```python
from build123d import *

# Parameters (mm, degrees)
BOSS_EXTRUDE1_DEPTH = 10
FILLET1_R           = 5
FILLET2_R           = 5
FILLET3_R           = 5


# Some blends are built 0.0001 mm under size
with BuildPart() as part:
    # Sketch1 → Boss-Extrude1 (new body)
    with BuildSketch(Plane.XY):
        Polygon((-40, -120.172625832), (-40, 169.827374168), (-25, 169.827374168), (-25, 219.827374168), (5, 219.827374168), (5, -170.172625832), (-25, -170.172625832), (-25, -120.172625832), align=None)
    extrude(amount=BOSS_EXTRUDE1_DEPTH)

    # Fillet1
    fillet1_edges = [part.edges().sort_by_distance(p)[0] for p in [
        (5, 24.827374168, 10),
        (5, 219.827374168, 5),
        (5, -170.172625832, 5),
        (5, 24.827374168, 0),
    ]]
    fillet(fillet1_edges, radius=FILLET1_R - 0.0001)  # a hair under: the kernel refuses the full size

    # Fillet2
    # the kernel refuses this fillet: 5 mm, written as the material it takes off along each edge
    with BuildSketch(Plane(origin=(5, -165.172625832, 5), x_dir=(0, -1, 0), z_dir=(0, 0, 1))) as fillet2_piece_1:
        with BuildLine():
            CenterArc((0.0001, -4.9999), 4.9999, 0, 90)
            Line((5, -4.9999), (5, 0))
            Line((5, 0), (0.0001, 0))
        make_face()
    revolve(axis=Axis((5, -165.172625832, 5), (1, 0, 0)), revolution_arc=90, mode=Mode.SUBTRACT)
    with BuildSketch(Plane(origin=(5, -165.172625832, 5), x_dir=(0, 0, 1), z_dir=(0, 1, 0))) as fillet2_piece_2:
        with BuildLine():
            CenterArc((0.0001, -4.9999), 4.9999, 0, 90)
            Line((5, -4.9999), (5, 0))
            Line((5, 0), (0.0001, 0))
        make_face()
    revolve(axis=Axis((5, -165.172625832, 5), (1, 0, 0)), revolution_arc=90, mode=Mode.SUBTRACT)
    with BuildSketch(Plane(origin=(5, -170.172625832, 0), x_dir=(0, 1, 0), z_dir=(-1, 0, 0))) as fillet2_piece_3:
        with BuildLine():
            CenterArc((FILLET2_R, -FILLET2_R), FILLET2_R, 90, 90)
            Line((0, -FILLET2_R), (0, 0))
            Line((0, 0), (FILLET2_R, 0))
        make_face()
    extrude(amount=42.5, mode=Mode.SUBTRACT)
    with BuildSketch(Plane(origin=(5, -170.172625832, 10), x_dir=(0, 1, 0), z_dir=(-1, 0, 0))) as fillet2_piece_4:
        with BuildLine():
            CenterArc((FILLET2_R, FILLET2_R), FILLET2_R, 180, 90)
            Line((0, FILLET2_R), (0, 0))
            Line((0, 0), (FILLET2_R, 0))
        make_face()
    extrude(amount=42.5, mode=Mode.SUBTRACT)

    # Fillet3
    # the kernel refuses this fillet: 5 mm, written as the material it takes off along each edge
    with BuildSketch(Plane(origin=(5, 214.827374168, 5), x_dir=(0, 0, -1), z_dir=(0, -1, 0))) as fillet3_piece_1:
        with BuildLine():
            CenterArc((0.0001, -4.9999), 4.9999, 0, 90)
            Line((5, -4.9999), (5, 0))
            Line((5, 0), (0.0001, 0))
        make_face()
    revolve(axis=Axis((5, 214.827374168, 5), (1, 0, 0)), revolution_arc=90, mode=Mode.SUBTRACT)
    with BuildSketch(Plane(origin=(5, 214.827374168, 5), x_dir=(0, 1, 0), z_dir=(0, 0, -1))) as fillet3_piece_2:
        with BuildLine():
            CenterArc((0.0001, -4.9999), 4.9999, 0, 90)
            Line((5, -4.9999), (5, 0))
            Line((5, 0), (0.0001, 0))
        make_face()
    revolve(axis=Axis((5, 214.827374168, 5), (1, 0, 0)), revolution_arc=90, mode=Mode.SUBTRACT)
    with BuildSketch(Plane(origin=(-37.5, 219.827374168, 0), x_dir=(0, 0, 1), z_dir=(1, 0, 0))) as fillet3_piece_3:
        with BuildLine():
            CenterArc((FILLET3_R, FILLET3_R), FILLET3_R, 180, 90)
            Line((0, FILLET3_R), (0, 0))
            Line((0, 0), (FILLET3_R, 0))
        make_face()
    extrude(amount=42.5, mode=Mode.SUBTRACT)
    with BuildSketch(Plane(origin=(-37.5, 219.827374168, 10), x_dir=(0, 0, -1), z_dir=(1, 0, 0))) as fillet3_piece_4:
        with BuildLine():
            CenterArc((FILLET3_R, -FILLET3_R), FILLET3_R, 90, 90)
            Line((0, -FILLET3_R), (0, 0))
            Line((0, 0), (FILLET3_R, 0))
        make_face()
    extrude(amount=42.5, mode=Mode.SUBTRACT)


solid = part.part
```
For this review, take the finished solid that the model builds, in its own axes (mm). A direction names the side the tool comes from. Round coordinates to 2 decimals unless told otherwise and drop trailing zeros. One line per item, written item: value. Start each with the question number.
(1) Wall thickness on line 1 (Y direction, x = -7.5, z = 4.5); line 2 (Y direction, x = -32, z = 1.5); line 3 (X direction, y = 33.5, z = 5.5): over which ranges is each line inside the solid? List them lowest first.
(2) Insertion check: pin 1 (3 mm diameter, centred on y = -134.5, z = 7, fed in from -X); pin 2 (1.5 mm diameter, centred on x = -15, z = 1.5, fed in from +Y); pin 3 (1 mm diameter, centred on x = -2, z = 3.5, fed in from -Y). Each pin has a flat end and moves straight along its axis. Give the tip position at first contact, or say it passes through.
(3) Machinability: for faces 1 (the flat face through (-25, -146, 5)), 2 (the flat face through (-33, 169.827, 5)), 3 (the cylindrical face through (-12.675, 219.826, 4.89)), which of the approach directions +Z, -Z, +X, -X, +Y, -Y give a long, thin tool a straight path to every point of the face, cutting with its end or side? Answer none if there is none.
Result:
1. line 1: -170.15 to 219.8
1. line 2: -120.17 to 169.83
1. line 3: -40 to 4.97
2. pin 1: x = -25
2. pin 2: y = 219
2. pin 3: y = -170.07
3. face 1: +Z, -Z, -X, -Y
3. face 2: +Z, -Z, -X, +Y
3. face 3: +X, -X, +Y
